Autodesk Fusion 360 part; units mm, degrees
sketch "スケッチ1" plane through (0, 0, 0) normal (0, 0, 1) x (1, 0, 0)
  line L0 (3.2, 13.7) -> (17.7, 13.7)
  line L1 (17.7, 13.7) -> (17.7, 3.2)
  line L2 (17.7, 3.2) -> (3.2, 3.2)
  line L3 (3.2, 3.2) -> (3.2, 13.7)
  line L4 (25.5, 13.2) -> (43, 13.2)
  line L5 (43, 13.2) -> (43, 3.2)
  line L6 (43, 3.2) -> (25.5, 3.2)
  line L7 (25.5, 3.2) -> (25.5, 13.2)
  line L8 (0, 0) -> (46, 0)
  line L9 (46, 0) -> (46, 16.9)
  line L10 (46, 16.9) -> (0, 16.9)
  line L11 (0, 16.9) -> (0, 0)
  line L12 (46, 0) -> (56, 0)
  line L13 (56, 0) -> (56, 46.9)
  line L14 (56, 46.9) -> (46, 46.9)
  line L15 (46, 46.9) -> (46, 0)
  line L16 (-19.2, 35.1) -> (-5, 35.1)
  line L17 (-5, 35.1) -> (-5, 24.9)
  line L18 (-5, 24.9) -> (-19.2, 24.9)
  line L19 (-19.2, 24.9) -> (-19.2, 35.1)
  line L20 (-19.2, -2.9) -> (-5, -2.9)
  line L21 (-5, -2.9) -> (-5, -13.1)
  line L22 (-5, -13.1) -> (-19.2, -13.1)
  line L23 (-19.2, -13.1) -> (-19.2, -2.9)
  line L24 (0, 16.9) -> (0, 38.3)
  line L25 (0, 38.3) -> (-21.2, 38.3)
  line L26 (-21.2, 38.3) -> (-21.2, -16.3)
  line L27 (-21.2, -16.3) -> (0, -16.3)
  line L28 (0, -16.3) -> (0, 0)
  dimension "d1" = 10.5
  dimension "d2" = 10
  dimension "d3" = 14.5
  dimension "d4" = 17.5
  dimension "d5" = 7.8
  dimension "d6" = 3.2
  dimension "d7" = 3.2
  dimension "d8" = 3.2
  dimension "d9" = 3.2
  dimension "d10" = 46
  dimension "d11" = 10
  dimension "d12" = 30
  dimension "d17" = 14.2
  dimension "d18" = 14.2
  dimension "d19" = 10.2
  dimension "d20" = 10.2
  dimension "d21" = 27.8
  dimension "d22" = 8
  dimension "d23" = 5
  dimension "d24" = 5
  dimension "d25" = 2
  dimension "d26" = 3.2
  dimension "d27" = 3.2
extrude "押し出し1" add sketch "スケッチ1" along normal blind 12
fillet "フィレット1" radius 1 8 edges at (3.2, 13.7, 6) (25.5, 13.2, 6) (3.2, 3.2, 6) (25.5, 3.2, 6) (43, 3.2, 6) (17.7, 3.2, 6) (43, 13.2, 6) (17.7, 13.7, 6)
Build history of the part. All positions in model axes, mm. A direction names the side the tool comes from. Give positions to 0.01 mm unless a question says otherwise; leave off trailing zeros. Loops run counter-clockwise (first coordinate to the right, second up) from the corner with the lowest first, then second, coordinate; pieces in that order, holes last. Notation, with made-up numbers: (28, 87.25) -> (62, 87.25) arc R31 ccw to (62, 118.25) -> close; hole circle Ø5 at (72, -16). An arc over 180 degrees is marked (long way). Answer in a Markdown table with one row per item.
Item 1: Slice it at C-C on y = 32. Write the cut outline in (x, z), plus the area to 3 significant figures.
Findings below:
| item | result |
|---|---|
| outline | (-21.2, 0) -> (-19.2, 0) -> (-19.2, 12) -> (-21.2, 12) -> close; (-5, 0) -> (0, 0) -> (0, 12) -> (-5, 12) -> close; (46, 0) -> (56, 0) -> (56, 12) -> (46, 12) -> close |
| area | 204 mm² |
Item 2: Tool access for faces 1 (the flat face through (34, 13.2, 6)), 2 (the flat face through (0, -8, 6)), 3 (the flat face through (0, 27, 6)): list every direction of +Z, -Z, +X, -X, +Y, -Y with a clear straight run to the whole face (end or side of a thin tool).
Findings below:
| item | result |
|---|---|
| face 1 | +Z, -Z |
| face 2 | +Z, -Z, +X, -Y |
| face 3 | +Z, -Z, +Y |
Item 3: Probe line 1 along X through (y, z) = (11, 2.5); line 2 along X through (y, z) = (28, 7.75); line 3 along Y through (x, z) = (-16.5, 8). List the from-to ranges inside material, lowest first. Write a range as [from, to].
Findings below:
| item | result |
|---|---|
| line 1 | x = [-21.2, 3.2], [17.7, 25.5], [43, 56] |
| line 2 | x = [-21.2, -19.2], [-5, 0], [46, 56] |
| line 3 | y = [-16.3, -13.1], [-2.9, 24.9], [35.1, 38.3] |
Item 4: Slice it at B-B on x = 28. Write the cut outline in (y, z), plus the area to 3 significant figures.
Findings below:
| item | result |
|---|---|
| outline | (0, 0) -> (3.2, 0) -> (3.2, 12) -> (0, 12) -> close; (13.2, 0) -> (16.9, 0) -> (16.9, 12) -> (13.2, 12) -> close |
| area | 82.8 mm² |
Item 5: Slice it at D-D on z = 10.25. Give the number of separate pieces and of enclosed holes in the cut face, plus the area to 3 significant figures.
Findings below:
| item | result |
|---|---|
| separate pieces | 1 |
| enclosed holes | 4 |
| area | 1,790 mm² |
Item 6: Slice it at A-A on y = 19. Write the cut outline in (x, z).
Findings below:
| item | result |
|---|---|
| outline | (-21.2, 0) -> (0, 0) -> (0, 12) -> (-21.2, 12) -> close; (46, 0) -> (56, 0) -> (56, 12) -> (46, 12) -> close |
Item 7: Mould opens along Y. For faces 4 (the flat face through (-12, 24.9, 6)), 5 (the flat face through (28, 0, 6)), 6 (the flat face through (34, 3.2, 6)), 7 (the flat face through (46, 32, 6)) say: pulls with the +Y half, pulls with the -Y half, needs draft (parallel to the pull), parting line crosses it, or undercut.
Findings below:
| item | result |
|---|---|
| face 4 | undercut |
| face 5 | pulls with the -Y half |
| face 6 | undercut |
| face 7 | needs draft |
Item 8: Flat gauge pins, fed straight in: P1, Ø2, axis at x = 9, z = 1.5, coming from the +Y side; P2, Ø6, axis at x = 30, z = 7, coming from the -Y side; P3, Ø1.5, axis at x = -11.5, z = 6.5, coming from the +Y side. Where does each tip first touch, or does it go through?
Findings below:
| item | result |
|---|---|
| P1 | stops at y = 16.9 |
| P2 | stops at y = 0 |
| P3 | stops at y = 38.3 |
